Work out the finished part from the listing and answer in its coordinate system (mm). Coordinates: 2 decimals unless noted, no trailing zeros. Write each loop counter-clockwise with the first axis right and the second up, starting at its lowest first coordinate (ties: lowest second). Pieces come first, ordered by that corner, then holes. Notation, with made-up numbers: (-24.75, 47) - (3.25, 47) arc R22 ccw to (3.25, 75) - close; hole circle Ø2 at (36.25, 45). An arc over 180 degrees is marked (long way). Use one line per item in the form item = value. Start each with the question number.
Item 1: Consider probe 1 along Z at (x, y) = (-24, -1); probe 2 along Y at (x, z) = (0, 5.25); probe 3 along X at (y, z) = (0, 8). Determine where each line is inside the solid, lowest interval first.
Item 2: A cutting plane is placed at D-D (z = 3.25). Write down the section's boundary in (x, y), then the cut area to 3 significant figures.
Item 3: A cutting plane is placed at B-B (y = 0). Write down the section's boundary in (x, z), then the cut area to 3 significant figures.
Item 4: Given pin 1 (4 mm diameter, centred on x = -1.5, z = 6, fed in from -Y); pin 2 (4 mm diameter, centred on x = 8.5, z = 6.5, fed in from -Y); pin 3 (2 mm diameter, centred on y = -23.5, z = 16, fed in from -X), each flat-ended and moving along its own axis, determine where each tip first touches the part or whether it passes through.
Item 5: A cutting plane is placed at C-C (z = 17.25). Write down the section's boundary in (x, y).
Item 6: A cutting plane is placed at A-A (x = 0). Write down the section's boundary in (y, z), then the cut area to 3 significant figures.
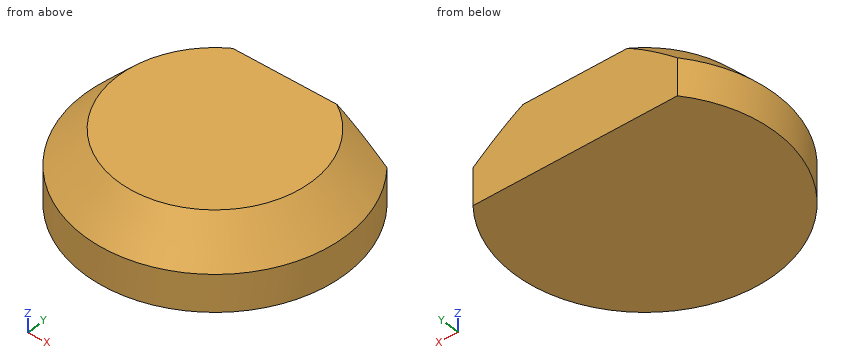
from build123d import *

# Parameters (mm, degrees)
F1_DEPTH = 2
F5_DEPTH = 19.589616
F7_DEPTH = 1.2


with BuildPart() as f1:
    # F0 (on Top) → F1 (new body)
    with BuildSketch(Plane.XY):
        with BuildLine():
            Line((27.229394, 21.99), (-27.229394, 21.99))
            ThreePointArc((-27.229394, 21.99), (0, -35), (27.229394, 21.99))
        make_face()
    extrude(amount=F1_DEPTH)

    # F2 (on Front) → F3 (revolve)
    with BuildSketch(Plane.XZ):
        Polygon((-35, 0), (-33.560254, 0), (-33.560254, 10), (-25.686589, 18.388616), (0, 18.388616), (0, 19.588616), (-26, 19.588616), (-35, 10), align=None)
    revolve(axis=Axis((0, 0, 12.407482), (0, 0, -1)))

    # F4 (on face) → F5 (cut, through all)
    with BuildSketch(Plane(origin=(0, 0, 0), x_dir=(1, 0, 0), z_dir=(0, 0, -1))):
        Polygon((27.229394, -21.99), (-25.352131, -21.99), (-27.229394, -21.99), (-27.229394, -37.239455), (27.229394, -37.239455), align=None)
    extrude(amount=-F5_DEPTH, mode=Mode.SUBTRACT)

    # F6 (on face) → F7 (join)
    with BuildSketch(Plane(origin=(0, 21.99, 0), x_dir=(-1, 0, 0), z_dir=(0, 1, 0))):
        Polygon((13.872271, 19.588616), (-13.872271, 19.588616), (-27.229394, 10), (-27.229394, 0), (27.229394, 0), (27.229394, 10), align=None)
    extrude(amount=-F7_DEPTH)


solid = f1.part
Answer:
q1.probe_1 = 0 to 2, 18.39 to 19.59
q1.probe_2 = -35 to -33.56, 20.79 to 21.99
q1.probe_3 = -35 to -33.56, 33.56 to 35
q2.outline = (-27.23, 21.99) arc R35 ccw (long way) to (27.23, 21.99) - close; hole (-26.35, 20.79) arc R33.56 ccw (long way) to (26.35, 20.79) - close
q2.area = 286 mm²
q3.outline = (-35, 0) - (35, 0) - (35, 10) - (26, 19.59) - (-26, 19.59) - (-35, 10) - close; hole (-33.56, 2) - (33.56, 2) - (33.56, 10) - (25.69, 18.39) - (-25.69, 18.39) - (-33.56, 10) - close
q3.area = 251 mm²
q4.pin_1 = -35
q4.pin_2 = -34.39
q4.pin_3 = -19.57
q5.outline = (-17.65, 21.99) arc R28.2 ccw (long way) to (17.65, 21.99) - close; hole (-16.84, 20.79) arc R26.76 ccw (long way) to (16.84, 20.79) - close
q6.outline = (-35, 0) - (21.99, 0) - (21.99, 19.59) - (-26, 19.59) - (-35, 10) - close; hole (-33.56, 2) - (20.79, 2) - (20.79, 18.39) - (-25.69, 18.39) - (-33.56, 10) - close
q6.area = 216 mm²
